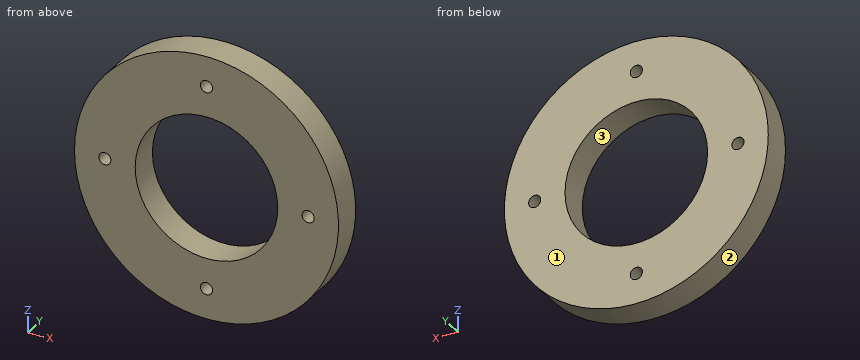
Autodesk Inventor part; units mm, degrees
ref_plane "YZ Plane" through (0, 0, 0) normal (1, 0, 0) x (0, 1, 0)
ref_plane "XZ Plane" through (0, 0, 0) normal (0, 1, 0) x (-1, 0, 0)
ref_plane "XY Plane" through (0, 0, 0) normal (0, 0, 1) x (1, 0, 0)
sketch "Sketch1" plane through (0, 0, 0) normal (0, 1, 0) x (-1, 0, 0)
  circle A0 centre (0, 0) radius 23.5
  circle A1 centre (0, 0) radius 43.5
  dimension "d0" = 47
  dimension "d1" = 87
extrude "Extrusion1" add sketch "Sketch1" along normal blind 10
sketch "Sketch2" plane through (0, 10, 0) normal (0, 1, 0) x (1, 0, 0)
  circle A0 centre (33.5, 0) radius 2
  point P0 (0, 0)
  dimension "d4" = 4
extrude "Extrusion2" cut sketch "Sketch2" against normal blind 10
mirror "Mirror1" about plane through (0, 0, 0) normal (1, 0, 0) of "Extrusion2"
sketch "Sketch3" plane through (0, 10, 0) normal (0, 1, 0) x (1, 0, 0)
  circle A0 centre (0, 33.5) radius 2
  circle A1 centre (0, -33.5) radius 2
  point P0 (0, 0)
  dimension "d7" = 4
  dimension "d8" = 4
extrude "Extrusion3" cut sketch "Sketch3" against normal blind 10
ref_plane "Work Plane1" through (0, 0, 0) normal (0, -1, 0) x (1, 0, 0)
properties part number "horizontal_lower_bearing_holder"
For this review, take the finished solid that the model builds, in its own axes (mm). Face numbers are marked on the shaded views. Coordinates: 2 decimals unless noted, no trailing zeros. Loops run counter-clockwise (first coordinate to the right, second up) from the corner with the lowest first, then second, coordinate; pieces in that order, holes last.
1. For line 1 (Z direction, x = 0, y = 2.25); line 2 (Z direction, x = -33.5, y = 6); line 3 (Z direction, x = -14.5, y = 3.5), list the stretches that pass through material, from the lowest coordinate up.
2. Add section A-A, the plane x = 0. Give the boundary of the cut face in (y, z).
3. Insertion check: P1, Ø2, axis at x = -8.5, y = 6, coming from the -Z side; P2, Ø2, axis at x = -18.5, y = 1.5, coming from the -Z side; P3, Ø2.5, axis at x = -33.5, z = 0, coming from the -Y side; P4, Ø1, axis at x = -8.5, y = 4.5, coming from the +Z side. Each pin has a flat end and moves straight along its axis. Give the tip position at first contact, or say it passes through.
4. Add section B-B, the plane z = 0. Give the boundary of the cut face in (x, y).
5. Add section D-D, the plane x = 33.5. Give the boundary of the cut face in (y, z).
6. Mouldability with a two-part tool opening along X and no side actions: class the marked faces 1, 2 and 3 as +X half, -X half, draft (parallel to the pull), parting line (faces both ways), or undercut.
7. Add section C-C, the plane y = 1.75. Give the boundary of the cut face in (x, z), then the cut area to 3 significant figures.
Result:
1. line 1: z = -43.5 to -35.5, -31.5 to -23.5, 23.5 to 31.5, 35.5 to 43.5
1. line 2: z = -27.75 to -2, 2 to 27.75
1. line 3: z = -41.01 to -18.49, 18.49 to 41.01
2. outline: (0, -43.5) - (10, -43.5) - (10, -35.5) - (0, -35.5) - close; (0, -31.5) - (10, -31.5) - (10, -23.5) - (0, -23.5) - close; (0, 23.5) - (10, 23.5) - (10, 31.5) - (0, 31.5) - close; (0, 35.5) - (10, 35.5) - (10, 43.5) - (0, 43.5) - close
3. P1: stops at z = -42.85
3. P2: stops at z = -39.82
3. P3: passes through
3. P4: stops at z = 42.76
4. outline: (-43.5, 0) - (-35.5, 0) - (-35.5, 10) - (-43.5, 10) - close; (-31.5, 0) - (-23.5, 0) - (-23.5, 10) - (-31.5, 10) - close; (23.5, 0) - (31.5, 0) - (31.5, 10) - (23.5, 10) - close; (35.5, 0) - (43.5, 0) - (43.5, 10) - (35.5, 10) - close
5. outline: (0, -27.75) - (10, -27.75) - (10, -2) - (0, -2) - close; (0, 2) - (10, 2) - (10, 27.75) - (0, 27.75) - close
6. face 1: draft
6. face 2: parting line
6. face 3: undercut
7. outline: circle Ø87 at (0, 0); hole circle Ø4 at (-33.5, 0); hole circle Ø47 at (0, 0); hole circle Ø4 at (0, -33.5); hole circle Ø4 at (0, 33.5); hole circle Ø4 at (33.5, 0)
7. area: 4,160 mm2
